Geometry check sheet. Reference: the model listing, model coordinates, mm. Coordinates: 2 decimals unless noted, no trailing zeros. Write each loop counter-clockwise with the first axis right and the second up, starting at its lowest first coordinate (ties: lowest second). Pieces come first, ordered by that corner, then holes. Notation, with made-up numbers: M -28.75,-3.75 L 27.25,-3.75 A14 cw 27.25,14.25 Z; hole C -7,45.5 d8. An arc over 180 degrees is marked long. Answer as a JSON object with one key per item and string values. Group by question number.
Autodesk Inventor part; units mm, degrees
ref_plane "YZ Plane" through (0, 0, 0) normal (1, 0, 0) x (0, 1, 0)
ref_plane "XZ Plane" through (0, 0, 0) normal (0, 1, 0) x (-1, 0, 0)
ref_plane "XY Plane" through (0, 0, 0) normal (0, 0, 1) x (1, 0, 0)
sketch "Sketch1" plane through (0, 0, 0) normal (0, 0, 1) x (1, 0, 0)
  line L0 (0, 0) -> (177.5, 0)
  line L1 (177.5, 0) -> (177.5, 135)
  line L2 (177.5, 135) -> (0, 135)
  line L3 (0, 135) -> (0, 0)
  dimension "d0" = 177.5
  dimension "d1" = 135
extrude "Extrusion1" add sketch "Sketch1" along normal blind 1
sketch "Sketch3" plane through (0, 0, 1) normal (0, 0, 1) x (1, 0, 0)
  line L0 (0, 0) -> (177.5, 0)
  line L1 (177.5, 0) -> (177.5, 135)
  line L2 (177.5, 135) -> (0, 135)
  line L3 (0, 135) -> (0, 0)
  line L4 (0, 128) -> (177.5, 128) construction
  line L5 (10, 135) -> (10, 0) construction
  line L6 (0, 88) -> (177.5, 88) construction
  line L7 (177.5, 70) -> (0, 70) construction
  line L8 (0, 30) -> (177.5, 30) construction
  line L9 (50, 135) -> (50, 0) construction
  line L10 (127.5, 135) -> (127.5, 0) construction
  line L11 (108.75, 135) -> (108.75, 0) construction
  line L12 (68.75, 135) -> (68.75, 0) construction
  line L13 (167.5, 135) -> (167.5, 0) construction
  line L14 (0, 7) -> (177.5, 7) construction
  point P0 (10, 128)
  point P1 (50, 128)
  point P2 (68.75, 128)
  point P3 (108.75, 128)
  point P4 (127.5, 128)
  point P5 (167.5, 128)
  point P6 (167.5, 88)
  point P7 (127.5, 88)
  point P8 (108.75, 88)
  point P9 (68.75, 88)
  point P10 (50, 88)
  point P11 (10, 88)
  point P12 (50, 30)
  point P13 (50, 70)
  point P14 (10, 70)
  point P15 (10, 30)
  point P16 (127.5, 30)
  point P17 (167.5, 30)
  point P18 (167.5, 70)
  point P19 (127.5, 70)
  point P20 (68.75, 70)
  point P21 (108.75, 70)
  point P22 (108.75, 30)
  point P23 (68.75, 30)
  point P24 (10, 7)
  point P25 (167.5, 7)
  point P26 (50, 7)
  point P27 (127.5, 7)
  dimension "d5" = 40
  dimension "d6" = 40
  dimension "d7" = 40
  dimension "d8" = 40
  dimension "d9" = 40
  dimension "d10" = 10
  dimension "d11" = 10
  dimension "d12" = 7
  dimension "d13" = 18
  dimension "d14" = 18.75
  dimension "d30" = 18.75
  dimension "d40" = 7
hole "Hole1" at (10, 128, 1) at (50, 128, 1) at (68.75, 128, 1) at (108.75, 128, 1) at (127.5, 128, 1) at (167.5, 128, 1) at (167.5, 88, 1) at (127.5, 88, 1) at (108.75, 88, 1) at (68.75, 88, 1) at (50, 88, 1) at (10, 88, 1) at (50, 30, 1) at (50, 70, 1) at (10, 70, 1) at (10, 30, 1) at (127.5, 30, 1) at (167.5, 30, 1) at (167.5, 70, 1) at (127.5, 70, 1) at (68.75, 70, 1) at (108.75, 70, 1) at (68.75, 30, 1) at (108.75, 30, 1) at (10, 7, 1) at (50, 7, 1) at (127.5, 7, 1) at (167.5, 7, 1) direction (0, 0, -1) diameter 4 end through all
sketch "Sketch4" plane through (0, 0, 1) normal (0, 0, 1) x (1, 0, 0)
  circle A0 centre (167.5, 70) radius 2
  circle A1 centre (127.5, 30) radius 2
  circle A2 centre (10, 70) radius 2
  circle A3 centre (50, 30) radius 2
  circle A4 centre (50, 88) radius 2
  circle A5 centre (108.75, 88) radius 2
  circle A6 centre (167.5, 88) radius 2
  circle A7 centre (127.5, 128) radius 2
  circle A8 centre (68.75, 128) radius 2
  circle A9 centre (10, 128) radius 2
  circle A10 centre (50, 128) radius 2
  circle A11 centre (108.75, 128) radius 2
  circle A12 centre (167.5, 128) radius 2
  circle A13 centre (127.5, 88) radius 2
  circle A14 centre (68.75, 88) radius 2
  circle A15 centre (10, 88) radius 2
  circle A16 centre (50, 70) radius 2
  circle A17 centre (10, 30) radius 2
  circle A18 centre (167.5, 30) radius 2
  circle A19 centre (127.5, 70) radius 2
  line L0 (10, 128) -> (50, 88) construction
  line L1 (68.75, 128) -> (108.75, 88) construction
  line L2 (50, 128) -> (10, 88) construction
  line L3 (68.75, 88) -> (108.75, 128) construction
  line L4 (127.5, 128) -> (167.5, 88) construction
  line L5 (167.5, 128) -> (127.5, 88) construction
  line L6 (127.5, 70) -> (167.5, 30) construction
  line L7 (167.5, 70) -> (127.5, 30) construction
  line L8 (10, 70) -> (50, 30) construction
  line L9 (50, 70) -> (10, 30) construction
  circle A20 centre (30, 108) radius 24
  circle A21 centre (88.75, 108) radius 24
  circle A22 centre (147.5, 108) radius 24
  circle A23 centre (147.5, 50) radius 24
  circle A24 centre (30, 50) radius 24
  circle A25 centre (68.75, 30) radius 2
  circle A26 centre (68.75, 70) radius 2
  circle A27 centre (108.75, 70) radius 2
  circle A28 centre (108.75, 30) radius 2
  line L10 (68.75, 70) -> (108.75, 30) construction
  line L11 (108.75, 70) -> (68.75, 30) construction
  circle A29 centre (88.75, 50) radius 24
  dimension "d22" = 48
  dimension "d23" = 48
  dimension "d24" = 48
  dimension "d25" = 48
  dimension "d26" = 48
  dimension "d29" = 48
extrude "Extrusion2" cut sketch "Sketch4" against normal blind 48 contours A20 | A21 | A22 | A23 | A24 | A29
equation "\"d27\" = d29"
properties part number "plate" material "ABS Plastic"
1) Section check C-C (y = 108). Record the cut outline in (x, z), then the cut area to 3 significant figures.
2) Section check A-A (y = 7). Record the cut outline in (x, z), then the cut area to 4 significant figures.
3) Section check B-B (x = 27). Record the cut outline in (y, z), then the cut area to 3 significant figures.
4) Draft check along X on faces 1 (the cylindrical face through (169.274, 87.077, 0.493)), 2 (the cylindrical face through (107.064, 86.925, 0.493)). Enter one of: +X half, -X half, draft (parallel to the pull), parting line (faces both ways), or undercut.
5) Go/stop test with a flat-tipped pin: pin 1 Ø3.5 at (x, y) = (50, 70) entering from +Z. Record where the tip stops, or that it passes through.
6) Section check D-D (x = 68.75). Record the cut outline in (y, z), then the cut area to 3 significant figures.
7) Material ranges on probe 1 along Y at (x, z) = (147, 0.7); probe 2 along Y at (x, z) = (71, 0.1); probe 3 along X at (y, z) = (58.5, 0.2), recorded low to high. Write a range as [from, to].
Entries:
{
 "1": {"outline": "M 0,0 L 6,0 L 6,1 L 0,1 Z; M 54,0 L 64.75,0 L 64.75,1 L 54,1 Z; M 112.75,0 L 123.5,0 L 123.5,1 L 112.75,1 Z; M 171.5,0 L 177.5,0 L 177.5,1 L 171.5,1 Z", "area": "33.5 mm^2"},
 "2": {"outline": "M 0,0 L 8,0 L 8,1 L 0,1 Z; M 12,0 L 48,0 L 48,1 L 12,1 Z; M 52,0 L 125.5,0 L 125.5,1 L 52,1 Z; M 129.5,0 L 165.5,0 L 165.5,1 L 129.5,1 Z; M 169.5,0 L 177.5,0 L 177.5,1 L 169.5,1 Z", "area": "161.5 mm^2"},
 "3": {"outline": "M 0,0 L 26.19,0 L 26.19,1 L 0,1 Z; M 73.81,0 L 84.19,0 L 84.19,1 L 73.81,1 Z; M 131.81,0 L 135,0 L 135,1 L 131.81,1 Z", "area": "39.8 mm^2"},
 "4": {"face 1": "undercut", "face 2": "undercut"},
 "5": {"pin 1": "through"},
 "6": {"outline": "M 0,0 L 28,0 L 28,1 L 0,1 Z; M 32,0 L 36.73,0 L 36.73,1 L 32,1 Z; M 63.27,0 L 68,0 L 68,1 L 63.27,1 Z; M 72,0 L 86,0 L 86,1 L 72,1 Z; M 90,0 L 94.73,0 L 94.73,1 L 90,1 Z; M 121.27,0 L 126,0 L 126,1 L 121.27,1 Z; M 130,0 L 135,0 L 135,1 L 130,1 Z", "area": "65.9 mm^2"},
 "7": {"probe 1": "[0, 26.01], [73.99, 84.01], [131.99, 135]", "probe 2": "[0, 33.85], [66.15, 91.85], [124.15, 135]", "probe 3": "[0, 7.56], [52.44, 66.31], [111.19, 125.06], [169.94, 177.5]"}
}
